Part print with two shaded views. Sizes in mm from the minimum x, y, z corner. Coordinates: 2 decimals unless noted, no trailing zeros. Order: outer loops, then holes, each group sorted by start corner. A loop starts at its lowest first (then second) coordinate and runs counter-clockwise, first axis right, second up. Notation, with made-up numbers: M -6,-3 L 47,-3 A20 ccw 47,29 Z; hole C -17.5,-1.5 d4. An arc over 180 degrees is marked long. Answer in a Markdown table with one row per item. Add a question column.
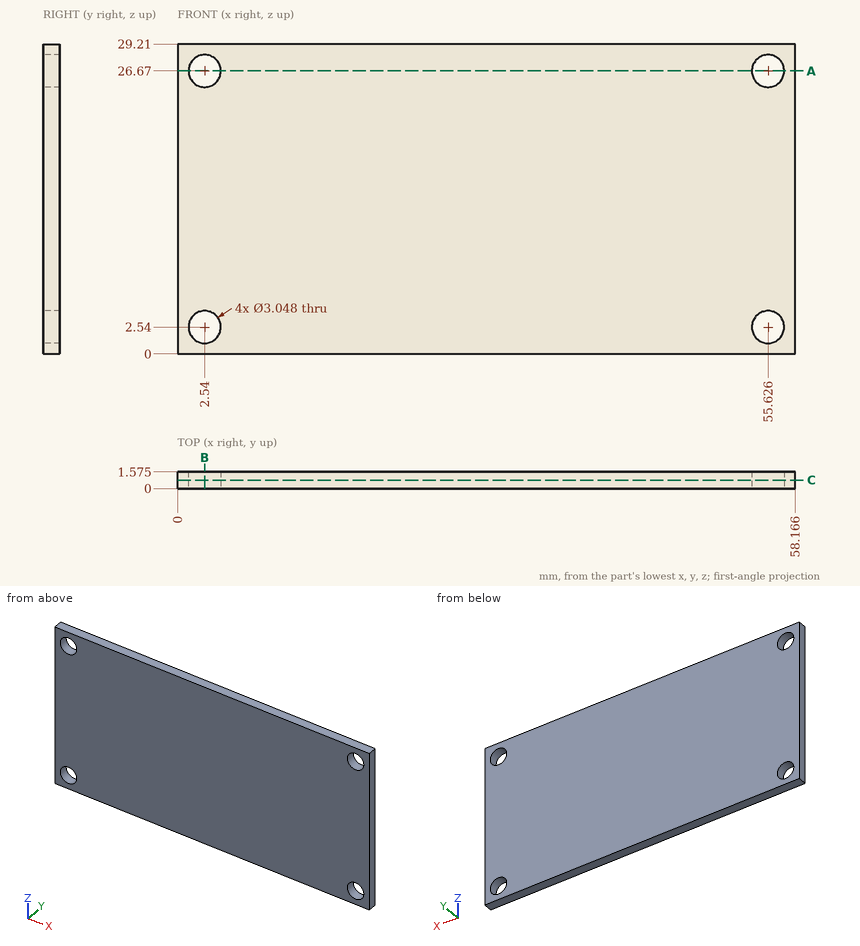
(1) Slice it at B-B (x = 2.54). List the corners of the cut face in (y, z) (1 decimal).
(2) Slice it at A-A (z = 26.67). State how many separate pieces and enclosed holes the cut face has, and give its area (3 significant figures).
(3) Slice it at C-C (y = 0.8). List the corners of the cut face in (x, z), and give its area (3 significant figures).
(4) Drop a flat-ended pin along its axis: P1, Ø1.8, axis at x = 55.626, z = 2.54, coming from the -Y side. Give the stop position or say it passes through.
(5) Wall check: line 1 (X direction, y = 1.25, z = 26.67); line 2 (Z direction, x = 2.54, y = 0.8); line 3 (Z direction, x = 3.5, y = 1.4). Give the ranges that are in metal, low to high.
Computed:
| question | item | result |
|---|---|---|
| 1 | outline | M 0,0 L 1.6,0 L 1.6,1 L 0,1 Z; M 0,4.1 L 1.6,4.1 L 1.6,25.1 L 0,25.1 Z; M 0,28.2 L 1.6,28.2 L 1.6,29.2 L 0,29.2 Z |
| 2 | separate pieces | 3 |
| 2 | enclosed holes | 0 |
| 2 | area | 82.0 mm^2 |
| 3 | outline | M 0,0 L 58.17,0 L 58.17,29.21 L 0,29.21 Z; hole C 2.54,2.54 d3.05; hole C 2.54,26.67 d3.05; hole C 55.63,2.54 d3.05; hole C 55.63,26.67 d3.05 |
| 3 | area | 1,670 mm^2 |
| 4 | P1 | passes through |
| 5 | line 1 | x = 0 to 1.02, 4.06 to 54.1, 57.15 to 58.17 |
| 5 | line 2 | z = 0 to 1.02, 4.06 to 25.15, 28.19 to 29.21 |
| 5 | line 3 | z = 0 to 1.36, 3.72 to 25.49, 27.85 to 29.21 |
